from build123d import *

# Parameters (mm, degrees)
F0_W      = 50.8
F0_H      = 50.8
F1_DEPTH  = 50.8
F3_T      = -5.08
F5_DEPTH  = 6.35
F6_R      = 21.461157
F7_DEPTH  = 6.35
F8_R      = 6.35
F8_R_2    = 7.078549
F9_DEPTH  = 6.35
F10_R     = 6.35
F11_DEPTH = 6.35


with BuildPart() as f1:
    # F0 (on Front) → F1 (new body)
    with BuildSketch(Plane.XZ):
        with Locations((-31.816838, -25.4)):
            Rectangle(F0_W, F0_H)
    extrude(amount=F1_DEPTH)

    # F3
    f3_openings = [f1.faces().sort_by_distance(p)[0] for p in [
        (-31.816838, -25.4, 0),
    ]]
    offset(amount=F3_T, openings=f3_openings)

    # F4 (on face) → F5 (cut)
    with BuildSketch(Plane(origin=(0, 0, 0), x_dir=(-1, 0, 0), z_dir=(0, 1, 0))):
        Polygon((49.197904, -15.436697), (31.878897, -5.365904), (14.497831, -15.329207), (14.435772, -35.363303), (31.754779, -45.434096), (49.135845, -35.470793), align=None)
    extrude(amount=-F5_DEPTH, mode=Mode.SUBTRACT)

    # F6 (on face) → F7 (cut)
    with BuildSketch(Plane(origin=(-57.216838, 0, 0), x_dir=(0, -1, 0), z_dir=(-1, 0, 0))):
        with Locations((25.4, -25.4)):
            Circle(F6_R)
    extrude(amount=-F7_DEPTH, mode=Mode.SUBTRACT)

    # F8 (on face) → F9 (join)
    with BuildSketch(Plane.YZ.offset(-6.416838)):
        with Locations((-38.671501, -12.8016)):
            Circle(F8_R)
        with Locations((-12.8016, -13.0683)):
            Circle(F8_R)
        with Locations((-25.4, -37.871402)):
            Circle(F8_R_2)
    extrude(amount=F9_DEPTH)

    # F10 (on face) → F11 (cut)
    with BuildSketch(Plane.XZ.offset(50.8)):
        with Locations((-31.816838, -37.871402)):
            Circle(F10_R)
        with Locations((-18.935701, -12.8016)):
            Circle(F10_R)
        with Locations((-45.072298, -13.0683)):
            Circle(F10_R)
    extrude(amount=-F11_DEPTH, mode=Mode.SUBTRACT)


solid = f1.part
CAD build for the part. Positions are in the model's coordinates, mm. A direction names the side the tool comes from. Give positions to 0.01 mm unless a question says otherwise; leave off trailing zeros. Write each loop counter-clockwise with the first axis right and the second up, starting at its lowest first coordinate (ties: lowest second). Pieces come first, ordered by that corner, then holes. Notation, with made-up numbers: M 2,77.25 L 17,77.25 A26 cw 17,109.25 Z; hole C 70.25,10 d9. An arc over 180 degrees is marked long. Put each result on its own line as item: value. Start each with the question number.
(1) Probe L1, parallel to Z at x = -56, y = -25; L2, parallel to X at y = -9.5, z = -4. List the from-to ranges inside material, lowest first.
(2) Flat gauge pins, fed straight in: pin 1 Ø10 at (x, z) = (-31.82, -37.87) entering from +Y; pin 2 Ø12 at (y, z) = (-27, -20.5) entering from -X; pin 3 Ø6.5 at (y, z) = (-13, -38) entering from +X; pin 4 Ø12 at (x, z) = (-26, -21.5) entering from +Y. Where does each tip first touch, or does it go through?
(3) Band-saw the part on D-D, the plane x = -40.5. Write the cut outline in (y, z), and give its area (3 significant figures).
(4) Mould opens along X. For faces 1 (the face through (-6.417, -25, -26)), 2 (the face through (-38, 0, -8)), 3 (the face through (-37, -5.08, -7)), 4 (the face through (-16.006, -48.296, -18.435)) say: +X half, -X half, draft (parallel to the pull), parting line (faces both ways), or undercut.
(5) Band-saw the part on A-A, the plane y = -25.4. Write the cut outline in (x, z).
(6) Band-saw the part on C-C, the plane z = -25.4. Write the cut outline in (x, y).
(7) Which spindle directions (+Z, -Z, +X, -X, +Y, -Y) get a long thin tool onto all of the face, cutting with end or side? Do faces 5 (the face through (-54.79, -20.75, -46.35)), 6 (the face through (-3.286, -6.936, -15.5)), 7 (the face through (-23.31, -2.5, -10.28)), 8 (the face through (-32, -25, -45.72)). Say none if no direction does.
(8) Band-saw the part on B-B, the plane z = -14.5. Give the number of separate pieces and of enclosed holes in the cut face, and give its area (3 significant figures).
Response values:
1. L1: z = -50.8 to -46.86, -3.94 to 0
1. L2: x = -57.22 to -52.14, -11.5 to -6.42
2. pin 1: passes through
2. pin 2: stops at x = -11.5
2. pin 3: stops at x = -6.42
2. pin 4: stops at y = -45.72
3. outline: M -50.8,-50.8 L 0,-50.8 L 0,-40.42 L -5.08,-40.42 L -5.08,-45.72 L -45.72,-45.72 L -45.72,-17.47 L -50.8,-17.47 Z; M -50.8,-8.66 L -45.72,-8.66 L -45.72,0 L -50.8,0 Z; M -5.08,-10.38 L 0,-10.38 L 0,0 L -5.08,0 Z
3. area: 525 mm2
4. face 1: +X half
4. face 2: draft
4. face 3: undercut
4. face 4: undercut
5. outline: M -57.22,-50.8 L -6.42,-50.8 L -6.42,-44.95 L -0.07,-44.95 L -0.07,-30.79 L -6.42,-30.79 L -6.42,0 L -11.5,0 L -11.5,-45.72 L -50.87,-45.72 L -50.87,-46.86 L -57.22,-46.86 Z; M -57.22,-3.94 L -52.14,-3.94 L -52.14,0 L -57.22,0 Z
6. outline: M -57.22,-50.8 L -6.42,-50.8 L -6.42,0 L -14.47,0 L -14.47,-5.08 L -11.5,-5.08 L -11.5,-45.72 L -50.87,-45.72 L -50.87,-46.86 L -57.22,-46.86 Z; M -57.22,-3.94 L -50.87,-3.94 L -50.87,-5.08 L -49.17,-5.08 L -49.17,0 L -57.22,0 Z
7. face 5: -X
7. face 6: +X
7. face 7: +Y
7. face 8: +Z
8. separate pieces: 4
8. enclosed holes: 0
8. area: 612 mm2
